Read the model definition and answer for the solid it produces. Units are mm, in the model's axes. Give positions to 0.01 mm unless a question says otherwise; leave off trailing zeros. Order: outer loops, then holes, each group sorted by start corner. A loop starts at its lowest first (then second) coordinate and runs counter-clockwise, first axis right, second up. Notation, with made-up numbers: M 4.25,5.25 L 29.25,5.25 A32 cw 29.25,36.25 Z; hole C 67.5,18.5 d5. An arc over 180 degrees is marked long. Write item = value, one per line. Start each with the question number.
from build123d import *

# Parameters (mm, degrees)
SKETCH1_R           = 1.651
BOSS_EXTRUDE1_DEPTH = 3.175


with BuildPart() as part:
    # Sketch1 → Boss-Extrude1 (new body)
    with BuildSketch(Plane.XY):
        with BuildLine():
            Line((-71.178896696, 3.175), (-50.858896696, 3.175))
            ThreePointArc((-50.858896696, 3.175), (-47.683896696, 0), (-50.858896696, -3.175))
            Line((-50.858896696, -3.175), (-71.178896696, -3.175))
            ThreePointArc((-71.178896696, -3.175), (-74.353896696, 0), (-71.178896696, 3.175))
        make_face()
        with Locations((-50.858896696, 0)):
            Circle(SKETCH1_R, mode=Mode.SUBTRACT)
        with Locations(Location((-71.178896696, 0, 0), (0, 0, 180))):
            Circle(SKETCH1_R, mode=Mode.SUBTRACT)
    extrude(amount=BOSS_EXTRUDE1_DEPTH)


solid = part.part
1) Find section B-B on z = 2.7. Determine the outline of the cut face in (x, y) (3 decimals), plus the area to 3 significant figures.
2) Find section A-A on y = 0. Determine the outline of the cut face in (x, z) (3 decimals).
3) For a pull along Y with two mould halves and no side action, classify faces 1 (the face through (-47.685, 0.07, 1.565)), 2 (the face through (-52.51, 0.07, 1.57)), 3 (the face through (-61, 0, 0)) as pulls with the +Y half, pulls with the -Y half, needs draft (parallel to the pull), parting line crosses it, or undercut.
4) Find the intervals of material crossed by probe 1 along X at (y, z) = (1, 0.9); probe 2 along X at (y, z) = (-0.5, 1.75); probe 3 along Y at (x, z) = (-71.5, 0.9), in increasing order. Write a range as [from, to].
5) Find section C-C on x = -71.5. Determine the outline of the cut face in (y, z) (3 decimals).
6) Find section D-D on y = -1.25. Determine the outline of the cut face in (x, z) (3 decimals).
Numbers:
q1.outline = M -71.179,-3.175 L -50.859,-3.175 A3.175 ccw -50.859,3.175 L -71.179,3.175 A3.175 ccw Z; hole C -71.179,0 d3.302; hole C -50.859,0 d3.302
q1.area = 144 mm2
q2.outline = M -74.354,0 L -72.83,0 L -72.83,3.175 L -74.354,3.175 Z; M -69.528,0 L -52.51,0 L -52.51,3.175 L -69.528,3.175 Z; M -49.208,0 L -47.684,0 L -47.684,3.175 L -49.208,3.175 Z
q3.face_1 = parting line crosses it
q3.face_2 = undercut
q3.face_3 = needs draft
q4.probe_1 = [-74.19, -72.49], [-69.87, -52.17], [-49.55, -47.85]
q4.probe_2 = [-74.31, -72.75], [-69.61, -52.43], [-49.29, -47.72]
q4.probe_3 = [-3.16, -1.62], [1.62, 3.16]
q5.outline = M -3.159,0 L -1.619,0 L -1.619,3.175 L -3.159,3.175 Z; M 1.619,0 L 3.159,0 L 3.159,3.175 L 1.619,3.175 Z
q6.outline = M -74.097,0 L -72.257,0 L -72.257,3.175 L -74.097,3.175 Z; M -70.1,0 L -51.937,0 L -51.937,3.175 L -70.1,3.175 Z; M -49.78,0 L -47.94,0 L -47.94,3.175 L -49.78,3.175 Z
